For this review, take the finished solid that the model builds, in its own axes (mm). A direction names the side the tool comes from. Round coordinates to 2 decimals unless told otherwise and drop trailing zeros. Write each loop counter-clockwise with the first axis right and the second up, starting at its lowest first coordinate (ties: lowest second). Pieces come first, ordered by that corner, then holes. Notation, with made-up numbers: (18.5, 51) - (44.5, 51) arc R18 cw to (44.5, 64) - close; hole circle Ø1 at (-30, 37). An arc over 180 degrees is marked (long way). One line per item, written item: value. Start each with the question number.
Q1. Add section B-B on z = 26. Write out the cut boundary in (x, y), and give its area (3 significant figures).
Q2. Tool access review of faces 5 (the face through (-2, -29, 0)), 6 (the face through (72, -113, 69.85)), 7 (the face through (-28.98, -130.52, 37.48)): name each direction out of +Z, -Z, +X, -X, +Y, -Y from which nothing blocks a thin tool from reaching the whole face with its end or side.
Q3. Clearance check with flat-ended pins moving along their axes: pin 1 Ø7.5 at (x, y) = (-108, -37.5) entering from -Z; pin 2 Ø4 at (x, y) = (66.5, 86) entering from -Z; pin 3 Ø20.5 at (x, y) = (0, -107.95) entering from +Z. State where each tip first meets the part, or that it passes through.
Q4. For probe 1 along X at (y, z) = (-107.95, -5.5) (3 decimals); probe 2 along Y at (x, z) = (0, 28.5); probe 3 along Z at (x, y) = (58, 53.5), list the stretches that pass through material, from the lowest coordinate up.
Q5. Add section C-C on y = -107.95. Write out the cut boundary in (x, z) (3 decimals), and give its area (3 significant figures).
Q6. Add section D-D on z = -143. Write out the cut boundary in (x, y) (1 decimal), and give its area (3 significant figures).
Q7. Mouldability with a two-part tool opening along X and no side actions: class faces 1 (the face through (5.86, -96.683, -5.916)), 2 (the face through (-57, 89, -12)), 3 (the face through (-64, 87, 0)), 4 (the face through (-107.118, -21.464, -5.916)) as +X half, -X half, draft (parallel to the pull), parting line (faces both ways), or undercut.
```python
from build123d import *

# Parameters (mm, degrees)
F0_R            = 139.7
F1_DEPTH        = 69.85
F2_T            = -6
F3_R            = 12.7
F3_R_2          = 6.375
F4_DEPTH        = 12
F4_COPIES_COUNT = 5
F6_R            = 4.7625
F7_DEPTH        = 266.7


# Not quite as in the source:
# - a pattern or mirror of a feature is missing from the dataset's text; its kind, count and spacing are read off the source's solid


with BuildPart() as f1:
    # F0 (on Top) → F1 (new body)
    with BuildSketch(Plane.XY):
        Circle(F0_R)
    extrude(amount=F1_DEPTH)

    # F2
    f2_openings = [f1.faces().sort_by_distance(p)[0] for p in [
        (0, 0, 69.85),
    ]]
    offset(amount=F2_T, openings=f2_openings)

    # F3 (on face) → F4 (join)
    with BuildSketch(Plane(origin=(0, 0, 0), x_dir=(1, 0, 0), z_dir=(0, 0, -1))):
        with Locations((0, 107.95)):
            Circle(F3_R)
        with Locations((0, 107.95)):
            Circle(F3_R_2, mode=Mode.SUBTRACT)
    f4 = extrude(amount=F4_DEPTH)

    # F4_copies: F4 ×5 about axis
    f4_copies_axis = Axis((0, 0, 0), (0, 0, 1))
    for i in range(1, F4_COPIES_COUNT):
        add(f4.rotate(f4_copies_axis, i * 360 / F4_COPIES_COUNT))

    # F6 (on face) → F7 (join)
    with BuildSketch(Plane(origin=(0, 0, 0), x_dir=(1, 0, 0), z_dir=(0, 0, -1))):
        Circle(F6_R)
    extrude(amount=F7_DEPTH)


solid = f1.part
```
Result set:
1. outline: circle Ø279.4 at (0, 0); hole circle Ø267.4 at (0, 0)
1. area: 5,150 mm^2
2. face 5: -Z
2. face 6: +Z, +X, -X, +Y, -Y
2. face 7: +Z
3. pin 1: stops at z = -12
3. pin 2: stops at z = 0
3. pin 3: stops at z = 6
4. probe 1: x = -12.7 to -6.375, 6.375 to 12.7
4. probe 2: y = -139.7 to -133.7, 133.7 to 139.7
4. probe 3: z = 0 to 6
5. outline: (-88.673, 0) - (-12.7, 0) - (-12.7, -12) - (-6.375, -12) - (-6.375, 0) - (6.375, 0) - (6.375, -12) - (12.7, -12) - (12.7, 0) - (88.673, 0) - (88.673, 69.85) - (78.883, 69.85) - (78.883, 6) - (-78.883, 6) - (-78.883, 69.85) - (-88.673, 69.85) - close
5. area: 2,470 mm^2
6. outline: circle Ø9.5 at (0, 0)
6. area: 71.3 mm^2
7. face 1: parting line
7. face 2: draft
7. face 3: undercut
7. face 4: undercut
